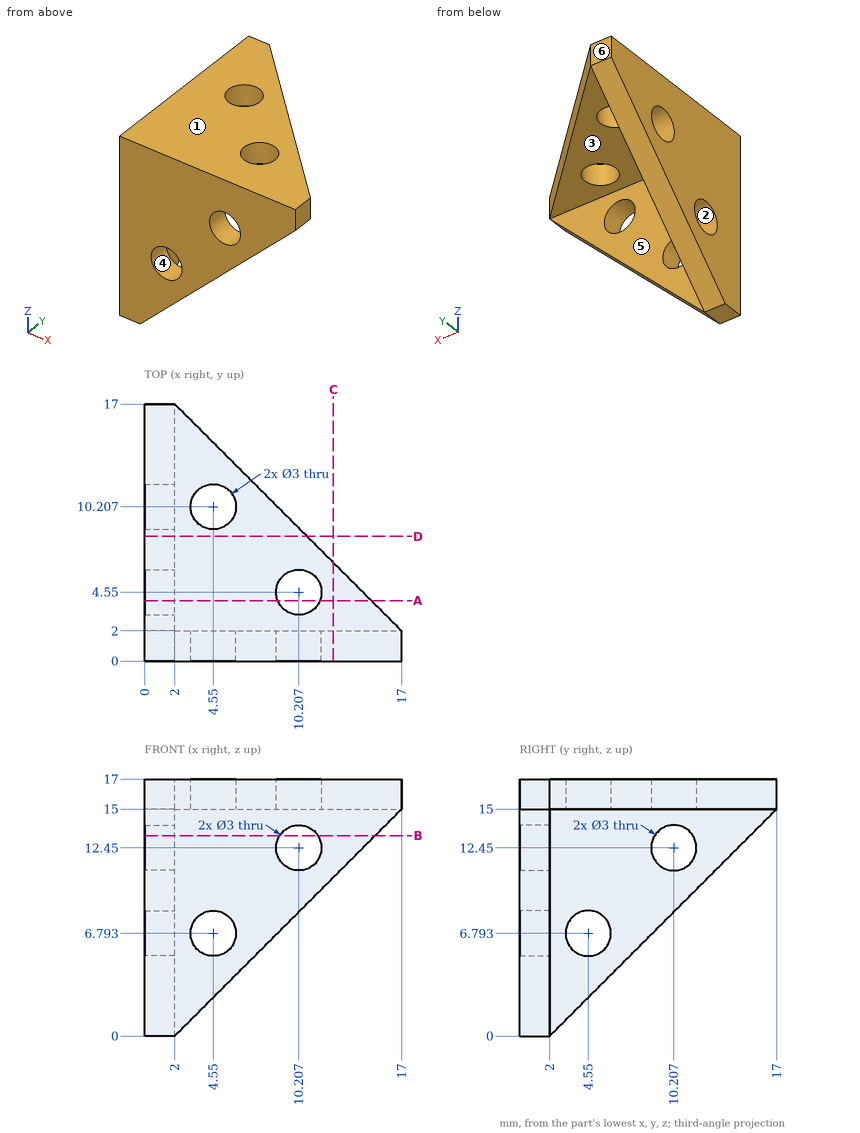
Could you check a few things on this drawing? It's one solid part, dimensions in mm from its lowest x, y, z. A direction names the side the tool comes from. Round coordinates to 2 decimals unless told otherwise and drop trailing zeros. Order: outer loops, then holes, each group sorted by start corner. A loop starts at its lowest first (then second) coordinate and runs counter-clockwise, first axis right, second up. Notation, with made-up numbers: M 32,50.5 L 63,50.5 A30 cw 63,83.5 Z; hole C 80.25,39 d2. An arc over 180 degrees is marked long. One line per question, with ' | ' between items. Start each with the question number.
(1) For P1, Ø7.5, axis at x = 7.5, y = 6, coming from the -Z side; P2, Ø8, axis at y = 14.5, z = 8.5, coming from the +X side, each with a flat end and sliding along its axis, tell me the tip position at first contact or that it passes through.
(2) Suppose I cut it at D-D on y = 8.25. List the corners of the cut face in (x, z) for me.
(3) Please list where these lines run through material, in increasing order: line 1 along Y through (x, z) = (6, 4.75); line 2 along Z through (x, y) = (6, 8).
(4) Thinking about a two-plate mould opening in Z: for the marked faces 1, 2, 3 and 4, which applies, +Z half, -Z half, draft (parallel to the pull), parting line (faces both ways), or undercut?
(5) Suppose I cut it at A-A on y = 4. List the corners of the cut face in (x, z) for me.
(6) Suppose I cut it at B-B on z = 13.25. List the corners of the cut face in (x, y) for me.
(7) Suppose I cut it at C-C on x = 12.5. List the corners of the cut face in (y, z) for me, then the cut area to 3 significant figures.
(8) For the marked faces 5 and 6, which set-ups out of +Z, -Z, +X, -X, +Y, -Y let a thin tool reach every point of the face, with its end or its side?
Geometry results:
1) P1: z = 15 | P2: x = 2
2) outline: M 0,6.25 L 2,6.25 L 2,15 L 10.75,15 L 10.75,17 L 0,17 Z
3) line 1: 0 to 2 | line 2: 15 to 17
4) face 1: +Z half | face 2: undercut | face 3: -Z half | face 4: undercut
5) outline: M 0,2 L 2,2 L 2,5.4 L 0,5.4 Z; M 0,8.19 L 2,8.19 L 2,15 L 8.81,15 L 8.81,17 L 0,17 Z; M 11.6,15 L 15,15 L 15,17 L 11.6,17 Z
6) outline: M 0,0 L 8.94,0 L 8.94,2 L 2,2 L 2,8.94 L 0,8.94 Z; M 0,11.48 L 2,11.48 L 2,15.25 L 0,15.25 Z; M 11.48,0 L 15.25,0 L 15.25,2 L 11.48,2 Z
7) outline: M 0,10.5 L 2,10.5 L 2,15 L 6.5,15 L 6.5,17 L 0,17 Z | area: 22.0 mm²
8) face 5: -Z, +X, +Y | face 6: +Z, -Z, +X, -X, +Y
